from build123d import *

# Parameters (mm, degrees)
F1_R     = 3.5
F1_R_2   = 2.75
F2_DEPTH = 5
F1_R_3   = 6
F3_DEPTH = 2
F4_SIZE  = 0.25


with BuildPart() as f2:
    # F1 (on Top) → F2 (new body)
    with BuildSketch(Plane.XY):
        Circle(F1_R)
        Circle(F1_R_2, mode=Mode.SUBTRACT)
    extrude(amount=F2_DEPTH)

    # F1 (on Top) → F3 (join)
    with BuildSketch(Plane.XY):
        Circle(F1_R_3)
        Circle(F1_R, mode=Mode.SUBTRACT)
    extrude(amount=F3_DEPTH)

    # F4
    f4_edges = [f2.edges().sort_by_distance(p)[0] for p in [
        (-3.5, 0, 5),
        (-3.5, 0, 2),
        (-6, 0, 2),
    ]]
    chamfer(f4_edges, length=F4_SIZE)


solid = f2.part
Can you work these out from the model? Positions are in its coordinate system, mm. A direction names the side the tool comes from. Give positions to 0.01 mm unless a question says otherwise; leave off trailing zeros. Loops run counter-clockwise (first coordinate to the right, second up) from the corner with the lowest first, then second, coordinate; pieces in that order, holes last. Notation, with made-up numbers: M 73,-38 L 132,-38 A23 cw 132,-4 Z; hole C 11,41.5 d6. An arc over 180 degrees is marked long. One line per item, written item: value.
1) Imagine slicing it at C-C on z = 0.6. Write out the boundary of the cut face in (x, y).
Geometry check:
outline: C 0,0 d12; hole C 0,0 d5.5
2) On a 3-axis mill with a long thin cutter (end or side, diameter ignored), from which of +Z, -Z, +X, -X, +Y, -Y can I reach the whole of each face in a straight line? I mean faces 1 (the face through (-6, 0, 1)), 2 (the face through (0, -4, 2)). Say none if no direction works.
Geometry check:
face 1: +Z, -Z
face 2: +Z
3) Thinking about a two-plate mould opening in X: for faces 3 (the face through (3, -1, 0)), 4 (the face through (3.233, -1.341, 3.482)), 5 (the face through (-0.596, -2.685, 2.465)), which applies, +X half, -X half, draft (parallel to the pull), parting line (faces both ways), or undercut?
Geometry check:
face 3: draft
face 4: parting line
face 5: undercut
4) Please list where these lines run through material, in increasing order: line 1 (Y direction, x = 0, z = 3.05); line 2 (Z direction, x = 3.75, y = 0.75); line 3 (Y direction, x = 0, z = 1.4).
Geometry check:
line 1: y = -3.5 to -2.75, 2.75 to 3.5
line 2: z = 0 to 2
line 3: y = -6 to -2.75, 2.75 to 6
5) I'm going to push a flat-ended pin straight in: pin 1 (1 mm diameter, centred on y = 0.5, z = 3, fed in from +X). Where does the tip first touch, or does it pass through?
Geometry check:
pin 1: stops at x = 3.5
6) Imagine slicing it at A-A on x = 0. Write out the boundary of the cut face in (y, z), and give its area (3 significant figures).
Geometry check:
outline: M -6,0 L -2.75,0 L -2.75,5 L -3.25,5 L -3.5,4.75 L -3.5,2.25 L -3.75,2 L -5.75,2 L -6,1.75 Z; M 2.75,0 L 6,0 L 6,1.75 L 5.75,2 L 3.75,2 L 3.5,2.25 L 3.5,4.75 L 3.25,5 L 2.75,5 Z
area: 17.4 mm²
7) Imagine slicing it at D-D on z = 3.8. Write out the boundary of the cut face in (x, y).
Geometry check:
outline: C 0,0 d7; hole C 0,0 d5.5
